Model file for the job. Use its own axes, mm. Give positions to 0.01 mm unless a question says otherwise; leave off trailing zeros. Loops run counter-clockwise (first coordinate to the right, second up) from the corner with the lowest first, then second, coordinate; pieces in that order, holes last. Notation, with made-up numbers: M 64,16 L 99,16 A32 ccw 99,49 Z; hole C 46.5,-29 d7. An arc over 180 degrees is marked long. Answer in a Markdown table with one row per item.
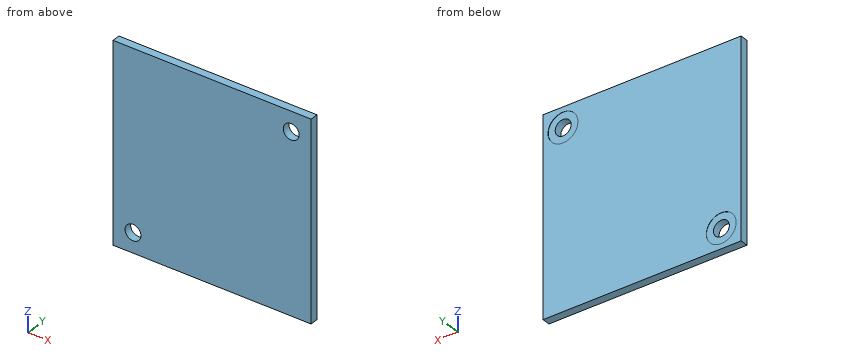
```python
from build123d import *

# Parameters (mm, degrees)
SKETCH1_W           = 39.8
SKETCH1_H           = 39.8
BOSS_EXTRUDE1_DEPTH = 1.6
SKETCH10_R          = 3
CUT_EXTRUDE6_DEPTH  = 0.05
SKETCH11_R          = 1.6
CUT_EXTRUDE7_DEPTH  = 1.6


with BuildPart() as part:
    # Sketch1 → Boss-Extrude1 (new body)
    with BuildSketch(Plane(origin=(0, 0, 0), x_dir=(1, 0, 0), z_dir=(0, 1, 0))):
        with Locations((-0.3, 0.3)):
            Rectangle(SKETCH1_W, SKETCH1_H)
    extrude(amount=BOSS_EXTRUDE1_DEPTH)

    # Sketch10 → Cut-Extrude6 (cut)
    with BuildSketch(Plane(origin=(0, 1.6, 0), x_dir=(1, 0, 0), z_dir=(0, 1, 0))):
        with Locations((-16.2, 16.2)):
            Circle(SKETCH10_R)
        with Locations((15.599994551, -15.586708083)):
            Circle(SKETCH10_R)
    extrude(amount=-CUT_EXTRUDE6_DEPTH, mode=Mode.SUBTRACT)

    # Sketch11 → Cut-Extrude7 (cut)
    with BuildSketch(Plane(origin=(0, 1.6, 0), x_dir=(1, 0, 0), z_dir=(0, 1, 0))):
        with Locations((-16.2, 16.2)):
            Circle(SKETCH11_R)
        with Locations((15.6, -15.6)):
            Circle(SKETCH11_R)
    extrude(amount=-CUT_EXTRUDE7_DEPTH, mode=Mode.SUBTRACT)


solid = part.part
```
Q1. Probe probe 1 along Z at (x, y) = (15.6, 0.6); probe 2 along Z at (x, y) = (16.5, 0.35). List the from-to ranges inside material, lowest first.
Reported:
| item | result |
|---|---|
| probe 1 | -20.2 to 14, 17.2 to 19.6 |
| probe 2 | -20.2 to 14.28, 16.92 to 19.6 |
Q2. Saw through at B-B (z = -16.2). Give the cut face in (x, y), and give its area (3 significant figures).
Reported:
| item | result |
|---|---|
| outline | M -20.2,0 L -17.8,0 L -17.8,1.55 L -19.2,1.55 L -19.2,1.6 L -20.2,1.6 Z; M -14.6,0 L 19.6,0 L 19.6,1.6 L -13.2,1.6 L -13.2,1.55 L -14.6,1.55 Z |
| area | 58.4 mm² |
Q3. Saw through at A-A (x = -16.2). Give the cut face in (y, z).
Reported:
| item | result |
|---|---|
| outline | M 0,-20.2 L 1.6,-20.2 L 1.6,-19.2 L 1.55,-19.2 L 1.55,-17.8 L 0,-17.8 Z; M 0,-14.6 L 1.55,-14.6 L 1.55,-13.2 L 1.6,-13.2 L 1.6,19.6 L 0,19.6 Z |
Q4. Drop flat-ended pins along their axis: pin 1 (3.5 mm diameter, centred on x = 15.6, z = 15.6, fed in from +Y); pin 2 (3 mm diameter, centred on x = -16.2, z = -16.2, fed in from +Y). Give the stop position or say it passes through.
Reported:
| item | result |
|---|---|
| pin 1 | y = 1.55 |
| pin 2 | through |
